```python
from build123d import *

# Parameters (mm, degrees)
SKETCH_W        = 215.9
SKETCH_H        = 38.1
PAD_DEPTH       = 114.3
SKETCH001_W     = 762
SKETCH001_H     = 19.05
POCKET_DEPTH    = 9.525
SKETCH003_W     = 76.2
SKETCH003_H     = 88.9
POCKET002_DEPTH = 19.05


with BuildPart() as part:
    # Sketch → Pad (new body)
    with BuildSketch(Plane.XY):
        Rectangle(SKETCH_W, SKETCH_H)
    extrude(amount=PAD_DEPTH)

    # Sketch001 (on Face6 of Pad) → Pocket (cut)
    with BuildSketch(Plane.XY.offset(114.3)):
        Rectangle(SKETCH001_W, SKETCH001_H)
    extrude(amount=-POCKET_DEPTH, mode=Mode.SUBTRACT)

    # Sketch003 → Pocket002 (cut)
    with BuildSketch(Plane.XZ.offset(19.05)):
        with Locations((0, 44.45)):
            Rectangle(SKETCH003_W, SKETCH003_H)
    extrude(amount=-POCKET002_DEPTH, mode=Mode.SUBTRACT)


solid = part.part
```
Input: part model. Units: mm. Frame: model coordinates. A direction names the side the tool comes from. Coordinates: 2 decimals unless noted, no trailing zeros. Loops run counter-clockwise (first coordinate to the right, second up) from the corner with the lowest first, then second, coordinate; pieces in that order, holes last. Notation, with made-up numbers: M 77,86 L 95,86 A15 cw 95,112 Z; hole C -5.5,30.5 d11. An arc over 180 degrees is marked long. Answer in a Markdown table with one row per item.
1. Section C-C, the plane x = 34. Output: boundary loops of the cut face in (y, z) (3 decimals).
Response:
| item | result |
|---|---|
| outline | M -19.05,88.9 L 0,88.9 L 0,0 L 19.05,0 L 19.05,114.3 L 9.525,114.3 L 9.525,104.775 L -9.525,104.775 L -9.525,114.3 L -19.05,114.3 Z |
2. Section D-D, the plane y = 6. Output: boundary loops of the cut face in (x, z) (3 decimals).
Response:
| item | result |
|---|---|
| outline | M -107.95,0 L 107.95,0 L 107.95,104.775 L -107.95,104.775 Z |
3. Reachability of faces 5 (the flat face through (-2, 0, 104.775)), 6 (the flat face through (107.95, 0, 56)), 7 (the flat face through (-1, 0, 45)) from +Z, -Z, +X, -X, +Y, -Y: full face, straight path, thin tool, end or side. Return the list, or none.
Response:
| item | result |
|---|---|
| face 5 | +Z, +X, -X |
| face 6 | +Z, -Z, +X, +Y, -Y |
| face 7 | -Z, -Y |
4. Draft query along Y for faces 1 (the flat face through (-107.95, 0, 56)), 2 (the flat face through (-2, 9.525, 110)), 3 (the flat face through (-2, 19.05, 56)), 4 (the flat face through (-2, -19.05, 94)). Return one class per face: pulls with the +Y half, pulls with the -Y half, needs draft (parallel to the pull), parting line crosses it, or undercut.
Response:
| item | result |
|---|---|
| face 1 | needs draft |
| face 2 | undercut |
| face 3 | pulls with the +Y half |
| face 4 | pulls with the -Y half |
5. Material intervals for line 1 (Y direction, x = -94.5, z = 106) (3 decimals); line 2 (X direction, y = -17, z = 69); line 3 (Y direction, x = -8, z = 79), sorted ascending.
Response:
| item | result |
|---|---|
| line 1 | y = -19.05 to -9.525, 9.525 to 19.05 |
| line 2 | x = -107.95 to -38.1, 38.1 to 107.95 |
| line 3 | y = 0 to 19.05 |
6. Section A-A, the plane y = -14. Output: boundary loops of the cut face in (x, z).
Response:
| item | result |
|---|---|
| outline | M -107.95,0 L -38.1,0 L -38.1,88.9 L 38.1,88.9 L 38.1,0 L 107.95,0 L 107.95,114.3 L -107.95,114.3 Z |
7. Section B-B, the plane z = 65. Output: boundary loops of the cut face in (x, y), then the cut area to 3 significant figures.
Response:
| item | result |
|---|---|
| outline | M -107.95,-19.05 L -38.1,-19.05 L -38.1,0 L 38.1,0 L 38.1,-19.05 L 107.95,-19.05 L 107.95,19.05 L -107.95,19.05 Z |
| area | 6,770 mm2 |
8. First-contact query: pin 1 (15 mm diameter, centred on x = -42.5, y = -0.5, fed in from +Z) (3 decimals). Flat tip, straight axial feed; report the tip coordinate or a pass-through.
Response:
| item | result |
|---|---|
| pin 1 | stops at z = 104.775 |
